The model under review builds one solid part; all positions refer to its coordinate system, in mm. Face numbers are marked on the shaded views. Coordinates: 2 decimals unless noted, no trailing zeros. Order: outer loops, then holes, each group sorted by start corner. A loop starts at its lowest first (then second) coordinate and runs counter-clockwise, first axis right, second up.
```python
from build123d import *

# Parameters (mm, degrees)
F0_R     = 2.25
F1_DEPTH = 8
F2_DEPTH = 1.2
F3_DEPTH = 5.8


with BuildPart() as f1:
    # F0 (on Right) → F1 (new body)
    with BuildSketch(Plane.YZ):
        with BuildLine():
            Line((-50, 0), (-48.8, 0))
            Line((-48.8, 0), (-48.8, 20.601839))
            ThreePointArc((-48.8, 20.601839), (-48.104502, 22.332091), (-46.404982, 23.099634))
            ThreePointArc((-46.404982, 23.099634), (-44.108069, 24.108069), (-43.099634, 26.404982))
            ThreePointArc((-43.099634, 26.404982), (-42.332091, 28.104502), (-40.601839, 28.8))
            Line((-40.601839, 28.8), (0, 28.8))
            Line((0, 28.8), (0, 30))
            Line((0, 30), (-46.396522, 30))
            Line((-46.396522, 30), (-46.703478, 30))
            ThreePointArc((-46.703478, 30), (-48.991931, 28.991931), (-50, 26.703478))
            Line((-50, 26.703478), (-50, 26.396522))
            Line((-50, 26.396522), (-50, 0))
        make_face()
        with Locations((-46.55, 26.55)):
            Circle(F0_R, mode=Mode.SUBTRACT)
    extrude(amount=F1_DEPTH)

    # F0 (on Right) → F2 (join)
    with BuildSketch(Plane.YZ):
        with BuildLine():
            Line((-48.8, 0), (0, 0))
            Line((0, 0), (0, 28.8))
            Line((0, 28.8), (-40.601839, 28.8))
            ThreePointArc((-40.601839, 28.8), (-42.332091, 28.104502), (-43.099634, 26.404982))
            ThreePointArc((-43.099634, 26.404982), (-44.108069, 24.108069), (-46.404982, 23.099634))
            ThreePointArc((-46.404982, 23.099634), (-48.104502, 22.332091), (-48.8, 20.601839))
            Line((-48.8, 20.601839), (-48.8, 0))
        make_face()
    extrude(amount=F2_DEPTH)

    # F0 (on Right) → F3 (join)
    with BuildSketch(Plane.YZ):
        with Locations((-46.55, 26.55)):
            Circle(F0_R)
    extrude(amount=F3_DEPTH)

    # F4: F1 across plane


with BuildPart() as f1_1:
    add(f1.part)
    add(f1.part.mirror(Plane.XZ))

    # F5: F1 across plane


with BuildPart() as f1_2:
    add(f1_1.part)
    add(f1_1.part.mirror(Plane.XY))


solid = f1_2.part
```
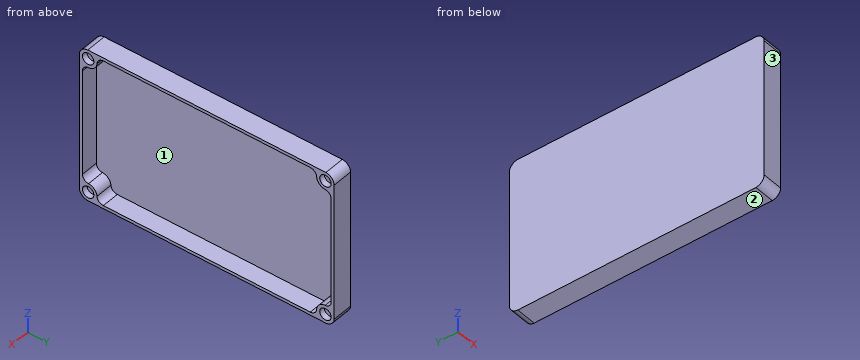
(1) Draft analysis for pull direction Y (two halves, no side actions). For the marked faces 1, 2 and 3, state which applies: released by +Y, released by -Y, zero draft, split by the parting line, or undercut.
A:
face 1: undercut
face 2: zero draft
face 3: released by -Y
(2) We need section A-A, the plane x = 2.75. Write out the cut boundary in (y, z).
A:
outline: (-50, -26.7) arc R3.45 ccw to (-46.7, -30) - (46.7, -30) arc R3.45 ccw to (50, -26.7) - (50, 26.7) arc R3.45 ccw to (46.7, 30) - (-46.7, 30) arc R3.45 ccw to (-50, 26.7) - close; hole (-48.8, -20.6) arc R2.5 ccw to (-46.4, -23.1) arc R3.45 cw to (-43.1, -26.4) arc R2.5 ccw to (-40.6, -28.8) - (40.6, -28.8) arc R2.5 ccw to (43.1, -26.4) arc R3.45 cw to (46.4, -23.1) arc R2.5 ccw to (48.8, -20.6) - (48.8, 20.6) arc R2.5 ccw to (46.4, 23.1) arc R3.45 cw to (43.1, 26.4) arc R2.5 ccw to (40.6, 28.8) - (-40.6, 28.8) arc R2.5 ccw to (-43.1, 26.4) arc R3.45 cw to (-46.4, 23.1) arc R2.5 ccw to (-48.8, 20.6) - close
(3) We need section B-B, the plane z = 16. Write out the cut boundary in (x, y), and give its area (3 significant figures).
A:
outline: (0, -50) - (8, -50) - (8, -48.8) - (1.2, -48.8) - (1.2, 48.8) - (8, 48.8) - (8, 50) - (0, 50) - close
area: 136 mm2
(4) We need section C-C, the plane y = -29.5. Write out the cut boundary in (x, z), and give its area (3 significant figures).
A:
outline: (0, -30) - (8, -30) - (8, -28.8) - (1.2, -28.8) - (1.2, 28.8) - (8, 28.8) - (8, 30) - (0, 30) - close
area: 88.3 mm2
(5) For pin 1 Ø4 at (y, z) = (-0.5, -14) entering from +X; pin 2 Ø2.5 at (y, z) = (46.55, 26.55) entering from +X, all flat-tipped, find the tip position at first contact; note any pin that passes through.
A:
pin 1: stops at x = 1.2
pin 2: stops at x = 5.8
(6) Wall thickness on probe 1 along Z at (x, y) = (6.5, 46.55); probe 2 along Y at (x, z) = (7.1, -26.55); probe 3 along Z at (x, y) = (7, 8): over which ranges is each line inside the solid? List them lowest first.
A:
probe 1: z = -30 to -28.8, -24.3 to -23.09, 23.09 to 24.3, 28.8 to 30
probe 2: y = -50 to -48.8, -44.3 to -43.09, 43.09 to 44.3, 48.8 to 50
probe 3: z = -30 to -28.8, 28.8 to 30
